Read the model definition and answer for the solid it produces. Units are mm, in the model's axes. A direction names the side the tool comes from. Coordinates: 2 decimals unless noted, no trailing zeros. Loops run counter-clockwise (first coordinate to the right, second up) from the corner with the lowest first, then second, coordinate; pieces in that order, holes last. Notation, with made-up numbers: (43, 26.25) - (69, 26.25) arc R21 cw to (69, 52.25) - close; hole circle Ø7 at (40.5, 85.5). An arc over 180 degrees is marked (long way). Use one line per item in the form item = value.
Autodesk Fusion 360 part; units mm, degrees
sketch "Sketch1" plane through (0, 0, 0) normal (0, 0, 1) x (1, 0, 0)
  line L0 (21, 7) -> (-21, 7)
  line L1 (-21, 7) -> (-21, -7)
  line L2 (-21, -7) -> (21, -7)
  line L3 (21, -7) -> (21, 7)
  line L4 (21, 7) -> (-21, -7) construction
  line L5 (-21, 7) -> (21, -7) construction
  line L6 (-16, 0) -> (16, 0) construction
  circle A0 centre (-16, 0) radius 2.35
  circle A1 centre (16, 0) radius 2.35
  dimension "d1" = 14
  dimension "d2" = 42
  dimension "d3" = 32
  dimension "d4" = 4.7
extrude "Extrude1" add sketch "Sketch1" along normal blind 3 contours L0 L1 L2 L3 | A0 | A1
sketch "Sketch2" plane through (0, 0, 3) normal (0, 0, 1) x (-1, 0, 0)
  line L0 (-21, 7) -> (-21, -7)
  line L1 (-21, -7) -> (21, -7)
  line L2 (21, -7) -> (21, 7)
  line L3 (21, 7) -> (-21, 7)
  line L4 (16, 0) -> (-16, 0) construction
  dimension "d7" = 32
hole "Hole1" at (-16, 0, 3) at (16, 0, 3) direction (0, 0, -1) diameter 3.3 depth 5 tip angle 180
sketch "Sketch3" plane through (0, 0, 0) normal (0, 0, -1) x (-1, 0, 0)
  circle A0 centre (16, 0) radius 1.65
  circle A1 centre (-16, 0) radius 1.65
  line L0 (-21, 6) -> (-21, -6)
  line L1 (-21, -6) -> (21, -6)
  line L2 (21, -6) -> (21, 6)
  line L3 (21, 6) -> (-21, 6)
  circle A2 centre (16, 0) radius 1.65
  circle A3 centre (-16, 0) radius 1.65
  line L4 (-21, 7) -> (-21, -7)
  line L5 (-21, -7) -> (21, -7)
  line L6 (21, -7) -> (21, 7)
  line L7 (21, 7) -> (-21, 7)
  line L8 (-12, -2) -> (12, -2)
  line L9 (12, -2) -> (12, 2)
  line L10 (12, 2) -> (-12, 2)
  line L11 (-12, 2) -> (-12, -2)
  line L12 (-12, -2) -> (12, 2) construction
  line L13 (12, -2) -> (-12, 2) construction
  dimension "d11" = 4
  dimension "d12" = 24
extrude "Extrude2" cut sketch "Sketch3" against normal blind 2 contours L8 L9 L10 L11
sketch "Sketch4" plane through (0, 0, 3) normal (0, 0, 1) x (-1, 0, 0)
  circle A0 centre (16, 0) radius 1.65
  circle A1 centre (-16, 0) radius 1.65
  line L0 (-21, 7) -> (-21, -7)
  line L1 (-21, -7) -> (21, -7)
  line L2 (21, -7) -> (21, 7)
  line L3 (21, 7) -> (-21, 7)
  line L4 (-9, -2.9) -> (9, -2.9)
  line L5 (9, -2.9) -> (9, 2.9)
  line L6 (9, 2.9) -> (-9, 2.9)
  line L7 (-9, 2.9) -> (-9, -2.9)
  line L8 (-9, -2.9) -> (9, 2.9) construction
  line L9 (9, -2.9) -> (-9, 2.9) construction
  dimension "d15" = 5.8
  dimension "d16" = 18
extrude "Extrude3" add sketch "Sketch4" along normal blind 1.4 contours L4 L5 L6 L7
fillet "Fillet1" radius 0.6 2 edges at (0, -2.9, 4.4) (0, 2.9, 4.4)
fillet "Fillet2" radius 1 4 edges at (-21, 7, 1.5) (21, 7, 1.5) (21, -7, 1.5) (-21, -7, 1.5)
Item 1: Which of the six approach directions +Z, -Z, +X, -X, +Y, -Y give full straight-line access (tool end or side, diameter ignored) to faces 1 (the flat face through (9, 0, 4)), 2 (the flat face through (-9, 0, 4)), 3 (the flat face through (0, 2, 1))?
Results below:
face_1 = +Z, +X, +Y, -Y
face_2 = +Z, -X, +Y, -Y
face_3 = -Z
Item 2: Find the intervals of material crossed by L1, parallel to X at y = 0, z = 2.4; L2, parallel to Y at x = 16, z = 1.55; L3, parallel to X at y = 0, z = 1.3, in increasing order.
Results below:
L1 = -21 to -17.65, -14.35 to 14.35, 17.65 to 21
L2 = -7 to -1.65, 1.65 to 7
L3 = -21 to -17.65, -14.35 to -12, 12 to 14.35, 17.65 to 21
Item 3: Each of these flat-tipped pins is pushed along its axis until it touches: P1, Ø0.7, axis at y = -1.5, z = 3.5, coming from the +X side; P2, Ø5.5, axis at x = -16, y = 0, coming from the +Z side; P3, Ø1.2, axis at x = 0, y = -0.5, coming from the -Z side; P4, Ø2.5, axis at x = 16, y = 0, coming from the +Z side. Where does it stop, or does it pass through?
Results below:
P1 = 9
P2 = 3
P3 = 2
P4 = through
Item 4: The part is cut by section C-C on z = 0.5. Give the vertices of the cut face in (x, y).
Results below:
outline = (-21, -6) arc R1 ccw to (-20, -7) - (20, -7) arc R1 ccw to (21, -6) - (21, 6) arc R1 ccw to (20, 7) - (-20, 7) arc R1 ccw to (-21, 6) - close; hole circle Ø3.3 at (-16, 0); hole (-12, -2) - (12, -2) - (12, 2) - (-12, 2) - close; hole circle Ø3.3 at (16, 0)
Item 5: The part is cut by section B-B on y = 0. Give the vertices of the cut face in (x, z).
Results below:
outline = (-21, 0) - (-17.65, 0) - (-17.65, 3) - (-21, 3) - close; (-14.35, 0) - (-12, 0) - (-12, 2) - (12, 2) - (12, 0) - (14.35, 0) - (14.35, 3) - (9, 3) - (9, 4.4) - (-9, 4.4) - (-9, 3) - (-14.35, 3) - close; (17.65, 0) - (21, 0) - (21, 3) - (17.65, 3) - close
Item 6: For a pull along X with two mould halves and no side action, classify faces 4 (the flat face through (12, 0, 1)), 5 (the cylindrical face through (20.699, -6.715, 1.521)), 6 (the flat face through (-21, 0, 1)), 7 (the cylindrical face through (17.6, 0.4, 1.5)) as +X half, -X half, draft (parallel to the pull), parting line (faces both ways), or undercut.
Results below:
face_4 = undercut
face_5 = +X half
face_6 = -X half
face_7 = undercut
Item 7: The part is cut by section D-D on x = -5. Give the vertices of the cut face in (y, z), plus the area to 3 significant figures.
Results below:
outline = (-7, 0) - (-2, 0) - (-2, 2) - (2, 2) - (2, 0) - (7, 0) - (7, 3) - (2.9, 3) - (2.9, 3.8) arc R0.6 ccw to (2.3, 4.4) - (-2.3, 4.4) arc R0.6 ccw to (-2.9, 3.8) - (-2.9, 3) - (-7, 3) - close
area = 42.0 mm²
Item 8: The part is cut by section A-A on x = 16. Give the vertices of the cut face in (y, z).
Results below:
outline = (-7, 0) - (-1.65, 0) - (-1.65, 3) - (-7, 3) - close; (1.65, 0) - (7, 0) - (7, 3) - (1.65, 3) - close
